CAD build for the part. Positions are in the model's coordinates, mm. A direction names the side the tool comes from. Coordinates: 2 decimals unless noted, no trailing zeros. Loops run counter-clockwise (first coordinate to the right, second up) from the corner with the lowest first, then second, coordinate; pieces in that order, holes last.
1) Saw through at B-B, the plane z = 92. Write the cut outline in (x, y).
2) Wall check: line 1 along X through (y, z) = (-4, 130.5); line 2 along Y through (x, z) = (28.5, 73). Give the ranges that are in metal, low to high.
3) Saw through at A-A, the plane x = -17. Write the cut outline in (y, z).
4) Two-plate mould, pull along X, no slides. Class faces 1 (the flat face through (-48, 24, 69)), 2 (the flat face through (49, -23, 69)), 3 (the flat face through (-1, -25, 69)), 4 (the flat face through (-1, -20, 69)): +X half, -X half, draft (parallel to the pull), parting line (faces both ways), or undercut.
5) Which spindle directions (+Z, -Z, +X, -X, +Y, -Y) get a long thin tool onto all of the face, cutting with end or side? Do faces 5 (the flat face through (45, 0, 69)), 6 (the flat face through (-50, 0, 69)). Say none if no direction does.
6) Saw through at C-C, the plane y = 14. Write the cut outline in (x, z).
```python
from build123d import *

# Parameters (mm, degrees)
F0_W     = 100
F0_H     = 50
F0_W_2   = 90
F0_H_2   = 40
F1_DEPTH = 140
F2_SIZE  = 3


with BuildPart() as f1:
    # F0 (on Top) → F1 (new body)
    with BuildSketch(Plane.XY):
        Rectangle(F0_W, F0_H)
        Rectangle(F0_W_2, F0_H_2, mode=Mode.SUBTRACT)
    extrude(amount=F1_DEPTH)

    # F2
    f2_edges = [f1.edges().sort_by_distance(p)[0] for p in [
        (50, -25, 70),
        (50, 25, 70),
        (-50, -25, 70),
        (-50, 25, 70),
    ]]
    chamfer(f2_edges, length=F2_SIZE)


solid = f1.part
```
Data:
1. outline: (-50, -22) - (-47, -25) - (47, -25) - (50, -22) - (50, 22) - (47, 25) - (-47, 25) - (-50, 22) - close; hole (-45, -20) - (45, -20) - (45, 20) - (-45, 20) - close
2. line 1: x = -50 to -45, 45 to 50
2. line 2: y = -25 to -20, 20 to 25
3. outline: (-25, 0) - (-20, 0) - (-20, 140) - (-25, 140) - close; (20, 0) - (25, 0) - (25, 140) - (20, 140) - close
4. face 1: -X half
4. face 2: +X half
4. face 3: draft
4. face 4: undercut
5. face 5: +Z, -Z
5. face 6: +Z, -Z, -X, +Y, -Y
6. outline: (-50, 0) - (-45, 0) - (-45, 140) - (-50, 140) - close; (45, 0) - (50, 0) - (50, 140) - (45, 140) - close
